Geometry check sheet. Reference: the model listing, model coordinates, mm. A direction names the side the tool comes from. Give positions to 0.01 mm unless a question says otherwise; leave off trailing zeros. Write each loop counter-clockwise with the first axis right and the second up, starting at its lowest first coordinate (ties: lowest second). Pieces come first, ordered by that corner, then holes. Notation, with made-up numbers: (40.25, -11.5) -> (57.25, -11.5) arc R20 ccw to (57.25, -3.5) -> close; hole circle Ø1 at (82, -11.75). An arc over 180 degrees is marked (long way). Write item = value, one per line. Start each with the question number.
1. Cross-section at B-B, the plane z = 7.25. Record the cut outline in (x, y), plus the area to 3 significant figures.
2. Thickness scan on line 1 along Z through (x, y) = (0, -1.6); line 2 along Z through (x, y) = (-2, 1.05); line 3 along X through (y, z) = (0.35, 4.5). Record the ranges inside material, lowest first.
3. Cross-section at C-C, the plane y = 1.2. Record the cut outline in (x, z).
4. Cross-section at A-A, the plane x = 0. Record the cut outline in (y, z), plus the area to 3 significant figures.
5. Cross-section at D-D, the plane z = 9.5. Record the cut outline in (x, y).
6. Depth check by flat-ended pin: P1, Ø1.7, axis at x = 4, z = 6.5, coming from the +Y side; P2, Ø0.8, axis at y = 2, z = 7, coming from the -X side; P3, Ø0.5, axis at y = 2, z = 4, coming from the +X side. Enter the tip coordinate at first touch or a pass-through.
7. Set-up check for faces 1 (the flat face through (-1.4, 2.5, 2.8)), 2 (the flat face through (3.1, 2, 5)), 3 (the flat face through (-4, 1.5, 5)): record each of +Z, -Z, +X, -X, +Y, -Y from which the full face is reachable in a straight line by a thin tool's end or side.
```python
from build123d import *

# Parameters (mm, degrees)
SKETCH2_W           = 6.2
SKETCH2_H           = 1
BOSS_EXTRUDE1_DEPTH = 10.5
CUT_EXTRUDE1_DEPTH  = 13.759800155


with BuildPart() as part:
    # Sketch2 → Boss-Extrude1 (new body)
    with BuildSketch(Plane.XY):
        Polygon((-3.1, 1.5), (-5.25, 1.5), (-5.25, -0.6), (-3.35, -2.5), (3.35, -2.5), (5.25, -0.6), (5.25, 1.5), (3.1, 1.5), align=None)
        with Locations((0, 2)):
            Rectangle(SKETCH2_W, SKETCH2_H)
    extrude(amount=BOSS_EXTRUDE1_DEPTH)

    # Sketch3 → Cut-Extrude1 (cut, through all)
    with BuildSketch(Plane(origin=(0, 2.5, 0), x_dir=(1, 0, 0), z_dir=(0, 1, 0))):
        with BuildLine():
            ThreePointArc((2.5, -5.25), (1.239388718, -3.078844638), (-1.271132484, -3.097275631))
            Line((-1.271132484, -3.097275631), (1.271132484, -7.402724369))
            ThreePointArc((1.271132484, -7.402724369), (2.171155362, -6.489388718), (2.5, -5.25))
        make_face()
        with BuildLine():
            Line((1.271132484, -7.402724369), (-1.271132484, -3.097275631))
            ThreePointArc((-1.271132484, -3.097275631), (-2.152724369, -6.521132484), (1.271132484, -7.402724369))
        make_face()
    extrude(amount=-CUT_EXTRUDE1_DEPTH, mode=Mode.SUBTRACT)


solid = part.part
```
Answers:
q1.outline = (-5.25, -0.6) -> (-3.35, -2.5) -> (-1.5, -2.5) -> (-1.5, 2.5) -> (-3.1, 2.5) -> (-3.1, 1.5) -> (-5.25, 1.5) -> close; (1.5, -2.5) -> (3.35, -2.5) -> (5.25, -0.6) -> (5.25, 1.5) -> (3.1, 1.5) -> (3.1, 2.5) -> (1.5, 2.5) -> close
q1.area = 29.6 mm^2
q2.line_1 = 0 to 2.75, 7.75 to 10.5
q2.line_2 = 0 to 3.75, 6.75 to 10.5
q2.line_3 = -5.25 to -2.38, 2.38 to 5.25
q3.outline = (-5.25, 0) -> (5.25, 0) -> (5.25, 10.5) -> (-5.25, 10.5) -> close; hole circle Ø5 at (0, 5.25)
q4.outline = (-2.5, 0) -> (2.5, 0) -> (2.5, 2.75) -> (-2.5, 2.75) -> close; (-2.5, 7.75) -> (2.5, 7.75) -> (2.5, 10.5) -> (-2.5, 10.5) -> close
q4.area = 27.5 mm^2
q5.outline = (-5.25, -0.6) -> (-3.35, -2.5) -> (3.35, -2.5) -> (5.25, -0.6) -> (5.25, 1.5) -> (3.1, 1.5) -> (3.1, 2.5) -> (-3.1, 2.5) -> (-3.1, 1.5) -> (-5.25, 1.5) -> close
q6.P1 = 1.5
q6.P2 = -3.1
q6.P3 = 3.1
q7.face_1 = +Z, -Z, +X, -X, +Y
q7.face_2 = +Z, -Z, +X, +Y
q7.face_3 = +Z, -Z, -X, +Y
